Autodesk Inventor part; units mm, degrees
ref_plane "YZ Plane" through (0, 0, 0) normal (1, 0, 0) x (0, 1, 0)
ref_plane "XZ Plane" through (0, 0, 0) normal (0, 1, 0) x (-1, 0, 0)
ref_plane "XY Plane" through (0, 0, 0) normal (0, 0, 1) x (1, 0, 0)
sketch "Esboço1" plane through (0, 0, 0) normal (1, 0, 0) x (0, 1, 0)
  line L0 (0, 0) -> (15, 0)
  line L1 (15, 0) -> (15, -5)
  line L2 (15, -5) -> (10, -5)
  line L3 (10, -30) -> (0, -30)
  line L4 (0, -30) -> (0, 0)
  line L5 (10, -5) -> (10, -8)
  arc A0 (10, -8) -> (10, -12) centre (10, -10) ccw
  line L6 (10, -12) -> (10, -30)
  point P0 (12.5, -5)
  point P1 (10, -6.5)
  dimension "d0" = 30
  dimension "d2" = 5
  dimension "d3" = 30
  dimension "d5" = 20
  dimension "d6" = 2
  dimension "d14" = 20
revolve "Revolução1" add sketch "Esboço1" angle 360 about axis through (0, 0, -30) along (0, 0, 1)
sketch "Esboço2" plane through (0, 0, -30) normal (0, 0, -1) x (-1, 0, 0)
  circle A0 centre (0, 0) radius 10
hole "Furo1" at (0, 0, -30) direction (0, 0, 1) diameter 10 end through all
thread "Rosca1"
chamfer "Chanfro1" distance 2 angle 45 1 edges at (0, -10, -30)
properties part number "3D Model"
Model file for the job. Use its own axes, mm. A direction names the side the tool comes from. Give positions to 0.01 mm unless a question says otherwise; leave off trailing zeros. Order: outer loops, then holes, each group sorted by start corner. A loop starts at its lowest first (then second) coordinate and runs counter-clockwise, first axis right, second up.
1) Wall check: probe 1 along X at (y, z) = (0, -23.5); probe 2 along Y at (x, z) = (0, -10). Give the ranges that are in metal, low to high.
2) Saw through at A-A, the plane x = 0. Write the cut outline in (y, z), then the cut area to 3 significant figures.
3) 3-axis set-ups, long thin cutter, end or side, ignore diameter. For faces 1 (the flat face through (10, 3, -5)), 2 (the cylindrical face through (0.66, -14.985, -2.535)): which of +Z, -Z, +X, -X, +Y, -Y reach the whole face in a straight line?
4) Pin check, flat tips, straight feed: pin 1 (10 mm diameter, centred on y = -10, z = -15, fed in from -X); pin 2 (1 mm diameter, centred on y = 0.5, z = -25, fed in from +X); pin 3 (3 mm diameter, centred on y = -10.5, z = -8.5, fed in from +X). Stop position of each tip, or through.
5) Saw through at D-D, the plane x = 11. Write the cut outline in (y, z).
6) Saw through at C-C, the plane z = -26. Write the cut outline in (x, y).
7) Mould opens along Y. For faces 3 (the cylindrical face through (-9.76, -2.17, -20.11)), 4 (the flat face through (5.2, -0.1, -30)), 5 (the cylindrical face through (4.88, -1.08, -14.79)) say: +Y half, -Y half, draft (parallel to the pull), parting line (faces both ways), or undercut.
Computed:
1. probe 1: x = -10 to -5, 5 to 10
1. probe 2: y = -8 to -5, 5 to 8
2. outline: (-15, -5) - (-10, -5) - (-10, -8) arc R2 cw to (-10, -12) - (-10, -28) - (-8, -30) - (-5, -30) - (-5, 0) - (-15, 0) - close; (5, -30) - (8, -30) - (10, -28) - (10, -12) arc R2 cw to (10, -8) - (10, -5) - (15, -5) - (15, 0) - (5, 0) - close
2. area: 333 mm2
3. face 1: -Z
3. face 2: +Z, -Z
4. pin 1: stops at x = -8.66
4. pin 2: stops at x = 10
4. pin 3: stops at x = 4.18
5. outline: (-10.2, -5) - (10.2, -5) - (10.2, 0) - (-10.2, 0) - close
6. outline: circle Ø20 at (0, 0); hole circle Ø10 at (0, 0)
7. face 3: parting line
7. face 4: draft
7. face 5: undercut
